The listing builds one solid part. Answer for the finished solid, in the listing's coordinates (mm). A direction names the side the tool comes from. Give positions to 0.01 mm unless a question says otherwise; leave off trailing zeros. Order: outer loops, then holes, each group sorted by start corner. A loop starts at its lowest first (then second) coordinate and runs counter-clockwise, first axis right, second up. Notation, with made-up numbers: (71.25, 41) - (88.25, 41) arc R29 ccw to (88.25, 73) - close; hole circle Ø7 at (84.5, 13.5). An arc over 180 degrees is marked (long way). Answer as a JSON object with one key per item and string values. Group by question number.
Q1. The mould has two halves that part along X. Classify faces 4 (the face through (253.005, 0, 72)), 5 (the face through (-190.4, -0.62, -14.14)), 6 (the face through (-11.575, 0.338, 764.878)): released by +X, released by -X, zero draft, split by the parting line, or undercut.
Q2. A cutting plane is placed at B-B, the plane x = 0. Give the vertices of the cut face in (y, z) (1 decimal).
Q3. Consider line 1 (X direction, y = 16, z = 35) (3 decimals); line 2 (Z direction, x = 0, y = 1.5); line 3 (X direction, y = 1.5, z = 366). Determine where each line is inside the solid, lowest interval first.
Q4. A cutting plane is placed at C-C, the plane z = 273.5. Give the vertices of the cut face in (x, y) (3 decimals), and give its area (3 significant figures).
Q5. Given pin 1 (24 mm diameter, centred on y = -11, z = 103, fed in from -X) (3 decimals); pin 2 (4 mm diameter, centred on x = -59, y = -1.5, fed in from +Z); pin 3 (8 mm diameter, centred on y = 10.5, z = 285, fed in from -X), each flat-ended and moving along its own axis, determine where each tip first touches the part or whether it passes through.
Q6. For faces 1 (the face through (11.493, 0.338, 761.874)), 2 (the face through (-2.611, -3.623, 11.505)), 3 (the face through (-253.005, 0, 70)), determine the directions among +Z, -Z, +X, -X, +Y, -Y from which every point of the face is accessible in a straight line to the end or side of a thin tool.
Q7. A cutting plane is placed at D-D, the plane x = 161. Give the vertices of the cut face in (y, z) (1 decimal).
from build123d import *

# Parameters (mm, degrees)
BOSS_EXTRUDE1_DEPTH = 24.125
CUT_EXTRUDE1_DEPTH  = 977.298322892


with BuildPart() as part:
    # Sketch1 → Revolve1 (revolve)
    with BuildSketch(Plane(origin=(0, 0, 0), x_dir=(1, 0, 0), z_dir=(0, 1, 0)), mode=Mode.PRIVATE) as revolve1_sk:
        Polygon((-250, 0), (250, 0), (250, 24.125), (209, 24.125), (186.495513174, 12.0625), (0, 12.0625), (-186.495513174, 12.0625), (-209, 24.125), (-250, 24.125), align=None)
    revolve(revolve1_sk.sketch.rotate(Axis((-250, 0, 0), (1, 0, 0)), 180), axis=Axis((-250, 0, 0), (1, 0, 0)))

    # Sketch3 → Boss-Extrude1 (add, symmetric)
    with BuildSketch(Plane(origin=(0, 0, 0), x_dir=(1, 0, 0), z_dir=(0, 1, 0))):
        with BuildLine():
            Line((-253.005, 0), (-253.005, -165.889796395))
            ThreePointArc((-253.005, -165.889796395), (0, -765.0675), (253.005, -165.889796395))
            Line((253.005, -165.889796395), (253.005, 0))
            Line((253.005, 0), (253.005, 24.125))
            Line((253.005, 24.125), (250, 24.125))
            Line((250, 24.125), (250, 0))
            Line((250, 0), (250, -167.113525722))
            ThreePointArc((250, -167.113525722), (0, -762.0625), (-250, -167.113525722))
            Line((-250, -167.113525722), (-250, 0))
            Line((-250, 0), (-250, 24.125))
            Line((-250, 24.125), (-253.005, 24.125))
            Line((-253.005, 24.125), (-253.005, 0))
        make_face()
    extrude(amount=BOSS_EXTRUDE1_DEPTH, both=True)

    # Sketch4 → Cut-Extrude1 (cut, through all)
    with BuildSketch(Plane.ZY.offset(253.005)):
        with BuildLine():
            ThreePointArc((-24.125, -2.4e-08), (-17.058951105, 17.058951087), (0, 24.125))
            Line((0, 24.125), (-24.125, 24.125))
            Line((-24.125, 24.125), (-24.125, -2.4e-08))
        make_face()
        with BuildLine():
            ThreePointArc((0, -24.125), (-17.058951087, -17.058951105), (-24.125, -2.4e-08))
            Line((-24.125, -2.4e-08), (-24.125, -24.125))
            Line((-24.125, -24.125), (0, -24.125))
        make_face()
    extrude(amount=-CUT_EXTRUDE1_DEPTH, mode=Mode.SUBTRACT)


solid = part.part
Reply:
{
 "1": {"face 4": "released by +X", "face 5": "undercut", "face 6": "split by the parting line"},
 "2": {"outline": "(-24.1, 762.1) - (24.1, 762.1) - (24.1, 765.1) - (-24.1, 765.1) - close; circle Ø24.1 at (0, 0)"},
 "3": {"line 1": "x = -253.005 to -250, 250 to 253.005", "line 2": "z = -11.97 to 11.97, 762.06 to 765.07", "line 3": "x = -349.99 to -346.96, 346.96 to 349.99"},
 "4": {"outline": "(-324.674, -24.125) - (-321.404, -24.125) - (-321.404, 24.125) - (-324.674, 24.125) - close; (321.404, -24.125) - (324.674, -24.125) - (324.674, 24.125) - (321.404, 24.125) - close", "area": "316 mm^2"},
 "5": {"pin 1": "stops at x = -253.005", "pin 2": "stops at z = 760.44", "pin 3": "stops at x = -330.86"},
 "6": {"face 1": "+Y, -Y", "face 2": "none", "face 3": "-Z, -X, +Y, -Y"},
 "7": {"outline": "(-24.1, 722.8) - (24.1, 722.8) - (24.1, 726.2) - (-24.1, 726.2) - close; circle Ø24.1 at (0, 0)"}
}
